Could you check a few things on this model? Use its own coordinates, in mm. Give positions to 0.01 mm unless a question says otherwise; leave off trailing zeros. Loops run counter-clockwise (first coordinate to the right, second up) from the corner with the lowest first, then second, coordinate; pieces in that order, holes last.
1. Imagine slicing it at C-C (y = 2.85). Count the separate pieces of the cut face and the enclosed holes in it, plus the area to 3 significant figures.
2. Imagine slicing it at A-A (z = 76). List the corners of the cut face in (x, y) for me, plus the area to 3 significant figures.
3. Imagine slicing it at B-B (x = 73). List the corners of the cut face in (y, z) for me.
4. I need wall thicknesses on line 1 along Z through (x, y) = (73, 2.1); line 2 along X through (y, z) = (2.7, -42); line 3 along X through (y, z) = (1, 21.5). Which ranges of each line are inside material? Lowest first, please.
5. For P1, Ø2.5, axis at x = 57, z = 52, coming from the +Y side, with a flat end and sliding along its axis, tell me the tip position at first contact or that it passes through.
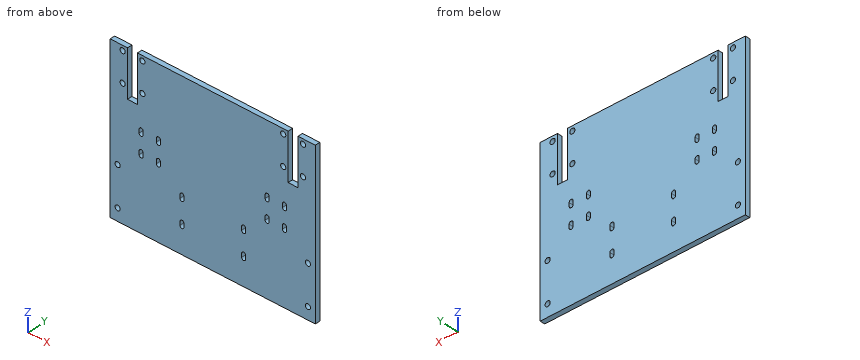
```python
from build123d import *

# Parameters (mm, degrees)
SKETCH1_W           = 166
SKETCH1_H           = 160
SKETCH1_R           = 2.1
BOSS_EXTRUDE1_DEPTH = 4
CUT_EXTRUDE1_DEPTH  = 5
SKETCH3_R           = 2.1
SKETCH3_W           = 8
SKETCH3_H           = 44
CUT_EXTRUDE2_DEPTH  = 10
SKETCH4_W           = 166
SKETCH4_H           = 28
CUT_EXTRUDE3_DEPTH  = 10
CUT_EXTRUDE4_DEPTH  = 5


with BuildPart() as part:
    # Sketch1 → Boss-Extrude1 (new body)
    with BuildSketch(Plane(origin=(0, 0, 0), x_dir=(1, 0, 0), z_dir=(0, 1, 0))):
        Rectangle(SKETCH1_W, SKETCH1_H)
        with Locations((-77, 74)):
            Circle(SKETCH1_R, mode=Mode.SUBTRACT)
        with Locations((-77, 10)):
            Circle(SKETCH1_R, mode=Mode.SUBTRACT)
        with Locations((77, 74)):
            Circle(SKETCH1_R, mode=Mode.SUBTRACT)
        with Locations((77, 10)):
            Circle(SKETCH1_R, mode=Mode.SUBTRACT)
        with Locations((-77, 42)):
            Circle(SKETCH1_R, mode=Mode.SUBTRACT)
        with Locations((77, 42)):
            Circle(SKETCH1_R, mode=Mode.SUBTRACT)
    extrude(amount=BOSS_EXTRUDE1_DEPTH)

    # Sketch2 → Cut-Extrude1 (cut)
    with BuildSketch(Plane(origin=(0, 4, 0), x_dir=(1, 0, 0), z_dir=(0, 1, 0))):
        with BuildLine():
            Line((-59.6, -24.5), (-59.6, -21.5))
            ThreePointArc((-59.6, -21.5), (-58, -19.9), (-56.4, -21.5))
            Line((-56.4, -21.5), (-56.4, -24.5))
            ThreePointArc((-56.4, -24.5), (-58, -26.1), (-59.6, -24.5))
        make_face()
        with BuildLine():
            Line((-45.6, -24.5), (-45.6, -21.5))
            ThreePointArc((-45.6, -21.5), (-44, -19.9), (-42.4, -21.5))
            Line((-42.4, -21.5), (-42.4, -24.5))
            ThreePointArc((-42.4, -24.5), (-44, -26.1), (-45.6, -24.5))
        make_face()
        with BuildLine():
            Line((-45.6, -8.5), (-45.6, -5.5))
            ThreePointArc((-45.6, -5.5), (-44, -3.9), (-42.4, -5.5))
            Line((-42.4, -5.5), (-42.4, -8.5))
            ThreePointArc((-42.4, -8.5), (-44, -10.1), (-45.6, -8.5))
        make_face()
        with BuildLine():
            Line((-59.6, -8.5), (-59.6, -5.5))
            ThreePointArc((-59.6, -5.5), (-58, -3.9), (-56.4, -5.5))
            Line((-56.4, -5.5), (-56.4, -8.5))
            ThreePointArc((-56.4, -8.5), (-58, -10.1), (-59.6, -8.5))
        make_face()
        with BuildLine():
            Line((59.6, -8.5), (59.6, -5.5))
            ThreePointArc((59.6, -5.5), (58, -3.9), (56.4, -5.5))
            Line((56.4, -5.5), (56.4, -8.5))
            ThreePointArc((56.4, -8.5), (58, -10.1), (59.6, -8.5))
        make_face()
        with BuildLine():
            Line((45.6, -8.5), (45.6, -5.5))
            ThreePointArc((45.6, -5.5), (44, -3.9), (42.4, -5.5))
            Line((42.4, -5.5), (42.4, -8.5))
            ThreePointArc((42.4, -8.5), (44, -10.1), (45.6, -8.5))
        make_face()
        with BuildLine():
            Line((45.6, -24.5), (45.6, -21.5))
            ThreePointArc((45.6, -21.5), (44, -19.9), (42.4, -21.5))
            Line((42.4, -21.5), (42.4, -24.5))
            ThreePointArc((42.4, -24.5), (44, -26.1), (45.6, -24.5))
        make_face()
        with BuildLine():
            Line((59.6, -24.5), (59.6, -21.5))
            ThreePointArc((59.6, -21.5), (58, -19.9), (56.4, -21.5))
            Line((56.4, -21.5), (56.4, -24.5))
            ThreePointArc((56.4, -24.5), (58, -26.1), (59.6, -24.5))
        make_face()
    extrude(amount=-CUT_EXTRUDE1_DEPTH, mode=Mode.SUBTRACT)

    # Sketch3 → Cut-Extrude2 (cut)
    with BuildSketch(Plane(origin=(0, 4, 0), x_dir=(1, 0, 0), z_dir=(0, 1, 0))):
        with Locations((-73, -76)):
            Circle(SKETCH3_R)
        with Locations((-57, -76)):
            Circle(SKETCH3_R)
        with Locations((-57, -52)):
            Circle(SKETCH3_R)
        with Locations((-73, -52)):
            Circle(SKETCH3_R)
        with Locations((73, -52)):
            Circle(SKETCH3_R)
        with Locations((57, -52)):
            Circle(SKETCH3_R)
        with Locations((57, -76)):
            Circle(SKETCH3_R)
        with Locations((73, -76)):
            Circle(SKETCH3_R)
        with Locations((-65, -64)):
            Rectangle(SKETCH3_W, SKETCH3_H)
        with Locations((65, -64)):
            Rectangle(SKETCH3_W, SKETCH3_H)
    extrude(amount=-CUT_EXTRUDE2_DEPTH, mode=Mode.SUBTRACT)

    # Sketch4 → Cut-Extrude3 (cut)
    with BuildSketch(Plane(origin=(0, 4, 0), x_dir=(1, 0, 0), z_dir=(0, 1, 0))):
        with Locations((0, 66)):
            Rectangle(SKETCH4_W, SKETCH4_H)
    extrude(amount=-CUT_EXTRUDE3_DEPTH, mode=Mode.SUBTRACT)

    # Sketch5 → Cut-Extrude4 (cut, through all)
    with BuildSketch(Plane(origin=(0, 4, 0), x_dir=(1, 0, 0), z_dir=(0, 1, 0))):
        with BuildLine():
            Line((-26.55, 28), (-26.55, 31))
            ThreePointArc((-26.55, 31), (-24.95, 32.6), (-23.35, 31))
            Line((-23.35, 31), (-23.35, 28))
            ThreePointArc((-23.35, 28), (-24.95, 26.4), (-26.55, 28))
        make_face()
        with BuildLine():
            Line((23.35, 28), (23.35, 31))
            ThreePointArc((23.35, 31), (24.95, 32.6), (26.55, 31))
            Line((26.55, 31), (26.55, 28))
            ThreePointArc((26.55, 28), (24.95, 26.4), (23.35, 28))
        make_face()
        with BuildLine():
            Line((23.35, 8), (23.35, 11))
            ThreePointArc((23.35, 11), (24.95, 12.6), (26.55, 11))
            Line((26.55, 11), (26.55, 8))
            ThreePointArc((26.55, 8), (24.95, 6.4), (23.35, 8))
        make_face()
        with BuildLine():
            Line((-26.55, 8), (-26.55, 11))
            ThreePointArc((-26.55, 11), (-24.95, 12.6), (-23.35, 11))
            Line((-23.35, 11), (-23.35, 8))
            ThreePointArc((-23.35, 8), (-24.95, 6.4), (-26.55, 8))
        make_face()
    extrude(amount=-CUT_EXTRUDE4_DEPTH, mode=Mode.SUBTRACT)


solid = part.part
```
Derived:
1. separate pieces: 1
1. enclosed holes: 24
1. area: 20,900 mm2
2. outline: (-83, 0) - (-75.1, 0) - (-75.1, 4) - (-83, 4) - close; (-70.9, 0) - (-69, 0) - (-69, 4) - (-70.9, 4) - close; (-61, 0) - (-59.1, 0) - (-59.1, 4) - (-61, 4) - close; (-54.9, 0) - (54.9, 0) - (54.9, 4) - (-54.9, 4) - close; (59.1, 0) - (61, 0) - (61, 4) - (59.1, 4) - close; (69, 0) - (70.9, 0) - (70.9, 4) - (69, 4) - close; (75.1, 0) - (83, 0) - (83, 4) - (75.1, 4) - close
2. area: 533 mm2
3. outline: (0, -52) - (4, -52) - (4, 49.9) - (0, 49.9) - close; (0, 54.1) - (4, 54.1) - (4, 73.9) - (0, 73.9) - close; (0, 78.1) - (4, 78.1) - (4, 80) - (0, 80) - close
4. line 1: z = -52 to 49.9, 54.1 to 73.9, 78.1 to 80
4. line 2: x = -83 to -79.1, -74.9 to 74.9, 79.1 to 83
4. line 3: x = -83 to -59.6, -56.4 to -45.6, -42.4 to 42.4, 45.6 to 56.4, 59.6 to 83
5. P1: passes through
